from build123d import *

# Parameters (mm, degrees)
SKETCH1_R                = 10
SKETCH1_R_2              = 2.1
SKETCH1_R_3              = 1.75
BOSS_EXTRUDE1_DEPTH      = 4
SKETCH2_R                = 9.05
CUT_EXTRUDE1_DEPTH       = 2.9
CHAMFER1_SIZE            = 1
BOSS_EXTRUDE2_DEPTH      = 2.9
BOSS_EXTRUDE2_DEPTH_BACK = 5.1
SKETCH3_R                = 2.1
CHAMFER2_SIZE            = 0.6
SKETCH4_R                = 3.1
CUT_EXTRUDE2_DEPTH       = 3
SKETCH5_R                = 2.1
CUT_EXTRUDE3_DEPTH       = 4
SKETCH6_R                = 0.625
CUT_EXTRUDE4_DEPTH       = 15.696938457
CIRPATTERN1_COUNT        = 3
CHAMFER3_SIZE            = 1
CHAMFER4_SIZE            = 1


with BuildPart() as part:
    # Sketch1 → Boss-Extrude1 (new, symmetric)
    with BuildSketch(Plane.XY):
        Circle(SKETCH1_R)
        with Locations((6, 0)):
            Circle(SKETCH1_R_2, mode=Mode.SUBTRACT)
        Circle(SKETCH1_R_3, mode=Mode.SUBTRACT)
        with Locations((0, -6)):
            Circle(SKETCH1_R_2, mode=Mode.SUBTRACT)
        with Locations((-6, 0)):
            Circle(SKETCH1_R_2, mode=Mode.SUBTRACT)
        with Locations((0, 6)):
            Circle(SKETCH1_R_2, mode=Mode.SUBTRACT)
    extrude(amount=BOSS_EXTRUDE1_DEPTH, both=True)

    # Sketch2 → Cut-Extrude1 (cut)
    with BuildSketch(Plane(origin=(0, 0, -4), x_dir=(-1, 0, 0), z_dir=(0, 0, -1))):
        Circle(SKETCH2_R)
    extrude(amount=-CUT_EXTRUDE1_DEPTH, mode=Mode.SUBTRACT)

    # Chamfer1
    # the kernel refuses this chamfer: 1 mm, written as the material it takes off along each edge
    with BuildSketch(Plane(origin=(0, 0, -4), x_dir=(-1, 0, 0), z_dir=(0, -1, 0))) as chamfer1_piece_1:
        Polygon((9.05 + CHAMFER1_SIZE, 0), (9.05, -CHAMFER1_SIZE), (9.05, 0), align=None)
    revolve(axis=Axis((0, 0, -4), (0, 0, -1)), mode=Mode.SUBTRACT)

    # Sketch3 → Boss-Extrude2 (add, two sides: drawn at the far end of the back side and taken through both)
    with BuildSketch(Plane(origin=(0, 0, -1.1), x_dir=(-1, 0, 0), z_dir=(0, 0, -1)).offset(-BOSS_EXTRUDE2_DEPTH_BACK)):
        with Locations((-6, 0)):
            Circle(SKETCH3_R)
        with Locations((0, -6)):
            Circle(SKETCH3_R)
        with Locations((6, 0)):
            Circle(SKETCH3_R)
        with Locations((0, 6)):
            Circle(SKETCH3_R)
    extrude(amount=BOSS_EXTRUDE2_DEPTH + BOSS_EXTRUDE2_DEPTH_BACK)

    # Chamfer2
    chamfer2_edges = [part.edges().sort_by_distance(p)[0] for p in [
        (8.1, 0, -4),
        (2.1, -6, -4),
        (-3.9, 0, -4),
        (2.1, 6, -4),
    ]]
    chamfer(chamfer2_edges, length=CHAMFER2_SIZE)

    # Sketch4 → Cut-Extrude2 (cut)
    with BuildSketch(Plane.XY.offset(4)):
        Circle(SKETCH4_R)
    extrude(amount=-CUT_EXTRUDE2_DEPTH, mode=Mode.SUBTRACT)

    # Sketch5 → Cut-Extrude3 (cut)
    with BuildSketch(Plane.XY.offset(4)):
        with Locations((0, 6.4)):
            Circle(SKETCH5_R)
        with Locations((5.542562584, -3.2)):
            Circle(SKETCH5_R)
        with Locations((-5.542562584, -3.2)):
            Circle(SKETCH5_R)
    extrude(amount=-CUT_EXTRUDE3_DEPTH, mode=Mode.SUBTRACT)

    # Sketch6 → Cut-Extrude4 (cut, through all)
    with BuildSketch(Plane.XY):
        with Locations((0, 6.4)):
            Circle(SKETCH6_R)
    cut_extrude4 = extrude(amount=-CUT_EXTRUDE4_DEPTH, mode=Mode.SUBTRACT)

    # CirPattern1: Cut-Extrude4 ×3 about axis
    cirpattern1_axis = Axis((0, 0, 0), (0, 0, 1))
    for i in range(1, CIRPATTERN1_COUNT):
        add(cut_extrude4.rotate(cirpattern1_axis, i * 360 / CIRPATTERN1_COUNT), mode=Mode.SUBTRACT)

    # Chamfer3
    chamfer3_edges = [part.edges().sort_by_distance(p)[0] for p in [
        (-0.625, 6.4, 0),
        (5.855062584, -2.658734123, 0),
        (-5.230062584, -3.741265877, 0),
    ]]
    chamfer(chamfer3_edges, length=CHAMFER3_SIZE)

    # Chamfer4
    # the kernel refuses this chamfer: 1 mm, written as the material it takes off along each edge
    with BuildSketch(Plane(origin=(0, 6.4, 4), x_dir=(1, 0, 0), z_dir=(0, -1, 0))) as chamfer4_piece_1:
        Polygon((2.1 + CHAMFER4_SIZE, 0), (2.1, -CHAMFER4_SIZE), (2.1, 0), align=None)
    revolve(axis=Axis((0, 6.4, 4), (0, 0, 1)), mode=Mode.SUBTRACT)
    with BuildSketch(Plane(origin=(5.542562584, -3.2, 4), x_dir=(1, 0, 0), z_dir=(0, -1, 0))) as chamfer4_piece_2:
        Polygon((2.1, -CHAMFER4_SIZE), (2.1 + CHAMFER4_SIZE, 0), (2.1, 0), align=None)
    revolve(axis=Axis((5.542562584, -3.2, 4), (0, 0, 1)), mode=Mode.SUBTRACT)
    with BuildSketch(Plane(origin=(-5.542562584, -3.2, 4), x_dir=(1, 0, 0), z_dir=(0, -1, 0))) as chamfer4_piece_3:
        Polygon((2.1 + CHAMFER4_SIZE, 0), (2.1, -CHAMFER4_SIZE), (2.1, 0), align=None)
    revolve(axis=Axis((-5.542562584, -3.2, 4), (0, 0, 1)), mode=Mode.SUBTRACT)
    with BuildSketch(Plane(origin=(0, 0, 4), x_dir=(1, 0, 0), z_dir=(0, -1, 0))) as chamfer4_piece_4:
        Polygon((10 - CHAMFER4_SIZE, 0), (10, -CHAMFER4_SIZE), (10, 0), align=None)
    revolve(axis=Axis((0, 0, 4), (0, 0, 1)), mode=Mode.SUBTRACT)
    with BuildSketch(Plane(origin=(0, 0, 4), x_dir=(1, 0, 0), z_dir=(0, -1, 0))) as chamfer4_piece_5:
        Polygon((3.1 + CHAMFER4_SIZE, 0), (3.1, -CHAMFER4_SIZE), (3.1, 0), align=None)
    revolve(axis=Axis((0, 0, 4), (0, 0, 1)), mode=Mode.SUBTRACT)


solid = part.part
Part model, mm, in its own coordinate system. A direction names the side the tool comes from. Round coordinates to 2 decimals unless told otherwise and drop trailing zeros. Use CSV: the item, a comma, the result in double quotes.
Item 1: Tool access for faces 5 (the flat face through (-5, -5, 0)), 6 (the flat face through (-6, 3, 4)), 7 (the cylindrical face through (-8.63, 2.72, -2.06)): list every direction of +Z, -Z, +X, -X, +Y, -Y with a clear straight run to the whole face (end or side of a thin tool).
Results list:
face 5,"+Z"
face 6,"+Z, +X, -X, +Y, -Y"
face 7,"-Z"
Item 2: Flat gauge pins, fed straight in: P1, Ø2, axis at x = -1, y = 6.5, coming from the +Z side; P2, Ø3.5, axis at x = -5.5, y = -2.5, coming from the +Z side; P3, Ø1, axis at x = 2, z = 1, coming from the +Y side. Where does each tip first touch, or does it go through?
Results list:
P1,"stops at z = 0"
P2,"stops at z = 3.35"
P3,"stops at y = 9.89"
Item 3: Wall check: L1, parallel to Y at x = 0, z = -1.75 (3 decimals); L2, parallel to Y at x = 0, z = 2.5; L3, parallel to Y at x = -7.75, z = -2.5. Give the ranges that are in metal, low to high.
Results list:
L1,"y = -10 to -9.05, -8.1 to -3.9, 3.9 to 5.775, 7.025 to 8.1, 9.05 to 10"
L2,"y = -10 to -3.1, 3.1 to 4.3, 8.5 to 10"
L3,"y = -6.32 to -4.67, -1.16 to 1.16, 4.67 to 6.32"
Item 4: Pull direction X, two halves, no side cores. Call faces 1 (the flat face through (0, -7, 4)), 2 (the cylindrical face through (1.617, -0.67, -0.065)), 3 (the cylindrical face through (-5.82, -1.12, 1.52)), 4 (the cylindrical face through (5.38, 8.43, -0.43)): pulls with the +X half, pulls with the -X half, needs draft (parallel to the pull), parting line crosses it, or undercut.
Results list:
face 1,"needs draft"
face 2,"undercut"
face 3,"undercut"
face 4,"parting line crosses it"
Item 5: Slice it at A-A, the plane x = 0. Count the separate pieces of the cut face and the enclosed holes in it, then the cut area to 3 significant figures.
Results list:
separate pieces,"3"
enclosed holes,"0"
area,"78.6 mm²"
